```python
from build123d import *

# Parameters (mm, degrees)
F1_DEPTH = 2
F2_R     = 2.25
F3_DEPTH = 25
F4_W     = 4
F4_H     = 2
F5_DEPTH = 10
F6_W     = 100
F6_H     = 5
F6_W_2   = 4
F6_H_2   = 6
F7_DEPTH = 13


with BuildPart() as f1:
    # F0 (on Top) → F1 (new body)
    with BuildSketch(Plane.XY):
        with BuildLine():
            Line((50, 28.866667), (194.856083, 112.499365))
            ThreePointArc((194.856083, 112.499365), (0, 225), (-194.856083, 112.499365))
            Line((-194.856083, 112.499365), (-50, 28.866667))
            Line((-50, 28.866667), (50, 28.866667))
        make_face()
    extrude(amount=F1_DEPTH)

    # F2 (on face) → F3 (cut)
    with BuildSketch(Plane.XY.offset(2)):
        with Locations((0, 52.116667)):
            Circle(F2_R)
        with Locations((0, 82.116667)):
            Circle(F2_R)
        with Locations((0, 112.116667)):
            Circle(F2_R)
        with Locations((0, 142.116667)):
            Circle(F2_R)
        with Locations((0, 172.116667)):
            Circle(F2_R)
        with Locations((0, 202.116667)):
            Circle(F2_R)
        with Locations((30, 52.116667)):
            Circle(F2_R)
        with Locations((30, 82.116667)):
            Circle(F2_R)
        with Locations((30, 112.116667)):
            Circle(F2_R)
        with Locations((30, 142.116667)):
            Circle(F2_R)
        with Locations((30, 172.116667)):
            Circle(F2_R)
        with Locations((30, 202.116667)):
            Circle(F2_R)
        with Locations((60, 52.116667)):
            Circle(F2_R)
        with Locations((60, 82.116667)):
            Circle(F2_R)
        with Locations((60, 112.116667)):
            Circle(F2_R)
        with Locations((60, 142.116667)):
            Circle(F2_R)
        with Locations((60, 172.116667)):
            Circle(F2_R)
        with Locations((60, 202.116667)):
            Circle(F2_R)
        with Locations((-30, 202.116667)):
            Circle(F2_R)
        with Locations((-30, 172.116667)):
            Circle(F2_R)
        with Locations((-30, 142.116667)):
            Circle(F2_R)
        with Locations((-30, 112.116667)):
            Circle(F2_R)
        with Locations((-30, 82.116667)):
            Circle(F2_R)
        with Locations((-30, 52.116667)):
            Circle(F2_R)
        with Locations((-60, 202.116667)):
            Circle(F2_R)
        with Locations((-60, 172.116667)):
            Circle(F2_R)
        with Locations((-60, 142.116667)):
            Circle(F2_R)
        with Locations((-60, 112.116667)):
            Circle(F2_R)
        with Locations((-60, 82.116667)):
            Circle(F2_R)
        with Locations((-60, 52.116667)):
            Circle(F2_R)
        with Locations((-90, 112.116667)):
            Circle(F2_R)
        with Locations((-90, 82.116667)):
            Circle(F2_R)
        with Locations((-90, 142.116667)):
            Circle(F2_R)
        with Locations((-90, 172.116667)):
            Circle(F2_R)
        with Locations((-120, 112.116667)):
            Circle(F2_R)
        with Locations((-120, 82.116667)):
            Circle(F2_R)
        with Locations((-120, 142.116667)):
            Circle(F2_R)
        with Locations((-120, 172.116667)):
            Circle(F2_R)
        with Locations((90, 112.116667)):
            Circle(F2_R)
        with Locations((90, 82.116667)):
            Circle(F2_R)
        with Locations((90, 142.116667)):
            Circle(F2_R)
        with Locations((90, 172.116667)):
            Circle(F2_R)
        with Locations((120, 112.116667)):
            Circle(F2_R)
        with Locations((120, 82.116667)):
            Circle(F2_R)
        with Locations((120, 142.116667)):
            Circle(F2_R)
        with Locations((120, 172.116667)):
            Circle(F2_R)
        with Locations((-150, 142.116667)):
            Circle(F2_R)
        with Locations((-150, 112.116667)):
            Circle(F2_R)
        with Locations((150, 142.116667)):
            Circle(F2_R)
        with Locations((150, 112.116667)):
            Circle(F2_R)
        with Locations((180, 112.116667)):
            Circle(F2_R)
        with Locations((-180, 112.116667)):
            Circle(F2_R)
    extrude(amount=-F3_DEPTH, mode=Mode.SUBTRACT)

    # F4 (on face) → F5 (join)
    with BuildSketch(Plane.XZ.offset(-28.866667)):
        with Locations((-9.5, 1)):
            Rectangle(F4_W, F4_H)
        with Locations((9.5, 1)):
            Rectangle(F4_W, F4_H)
    extrude(amount=F5_DEPTH)

    # F6 (on face) → F7 (join)
    with BuildSketch(Plane(origin=(0, 0, 0), x_dir=(1, 0, 0), z_dir=(0, 0, -1))):
        with Locations((0, -31.366667)):
            Rectangle(F6_W, F6_H)
        with Locations((-9.5, -21.866667)):
            Rectangle(F6_W_2, F6_H_2)
        with Locations((9.5, -21.866667)):
            Rectangle(F6_W_2, F6_H_2)
    extrude(amount=F7_DEPTH)


solid = f1.part
```
Could you check a few things on this model? Use its own coordinates, in mm. A direction names the side the tool comes from. Round coordinates to 2 decimals unless told otherwise and drop trailing zeros. Loops run counter-clockwise (first coordinate to the right, second up) from the corner with the lowest first, then second, coordinate; pieces in that order, holes last. Notation, with made-up numbers: M 0,0.5 L 8,0.5 A28 ccw 8,18.5 Z; hole C 81,-30 d2. An arc over 180 degrees is marked long. Write item = value, one per line.
1. I want a section at B-B, the plane y = 121. Write out the boundary of the cut face in (x, z), and give its area (3 significant figures).
Results below:
outline = M -189.69,0 L 189.69,0 L 189.69,2 L -189.69,2 Z
area = 759 mm²
2. Will these pins go through, and if not, where does the flat tip stop? P1, Ø1.5, axis at y = 31.5, z = -8, coming from the -X side; P2, Ø4, axis at x = -122.5, y = 133, coming from the -Z side; P3, Ø6, axis at x = -150, y = 142.12, coming from the +Z side; P4, Ø8, axis at y = 24.5, z = -5.5, coming from the +X side.
Results below:
P1 = -50
P2 = 0
P3 = 2
P4 = 11.5
3. Which directions (+Z, -Z, +X, -X, +Y, -Y) give clear straight access to the entire face, cutting with the end or side of a thin tool? Please do faces 1 (the face through (11.5, 22, -6)), 2 (the face through (7.5, 22, -6)), 3 (the face through (-3, 123, 2)), 4 (the face through (-11.5, 22, -6)).
Results below:
face_1 = +Z, -Z, +X, -Y
face_2 = +Z, -Z, -Y
face_3 = +Z, +X, -X, +Y, -Y
face_4 = +Z, -Z, -X, -Y
4. I want a section at C-C, the plane x = -129.5. Write out the boundary of the cut face in (y, z), and give its area (3 significant figures).
Results below:
outline = M 74.77,0 L 184,0 L 184,2 L 74.77,2 Z
area = 218 mm²
5. Thinking about a two-plate mould opening in X: for faces 5 (the face through (-1, 33.867, -6)), 6 (the face through (-7.5, 22, -6)), 7 (the face through (-123.442, 71.268, 0.986)), which applies, +X half, -X half, draft (parallel to the pull), parting line (faces both ways), or undercut?
Results below:
face_5 = draft
face_6 = undercut
face_7 = -X half
6. I need wall thicknesses on probe 1 along Y at (x, z) = (-90, 1.35); probe 2 along Z at (x, y) = (55.5, 178.5); probe 3 along X at (y, z) = (55, 1). Which ranges of each line are inside material? Lowest first, please.
Results below:
probe_1 = 51.96 to 79.87, 84.37 to 109.87, 114.37 to 139.87, 144.37 to 169.87, 174.37 to 206.22
probe_2 = 0 to 2
probe_3 = -95.26 to 95.26
7. I want a section at A-A, the plane z = -5.5. Write out the boundary of the cut face in (x, y), and give its area (3 significant figures).
Results below:
outline = M -50,28.87 L 50,28.87 L 50,33.87 L -50,33.87 Z; M -11.5,18.87 L -7.5,18.87 L -7.5,24.87 L -11.5,24.87 Z; M 7.5,18.87 L 11.5,18.87 L 11.5,24.87 L 7.5,24.87 Z
area = 548 mm²
